Can you work these out from the model? Positions are in its coordinate system, mm. A direction names the side the tool comes from. Give positions to 0.01 mm unless a question says otherwise; leave off trailing zeros. Order: outer loops, then holes, each group sorted by start corner. A loop starts at its lowest first (then second) coordinate and runs counter-clockwise, first axis right, second up. Notation, with made-up numbers: M -36.5,75 L 18.5,75 A17 ccw 18.5,101 Z; hole C 62,50.5 d7. An arc over 180 degrees is marked long. Answer as a JSON object with one key per item and string values.
```python
from build123d import *

# Parameters (mm, degrees)
EXTRUDE_1_DEPTH          = 9.7
CUT_EXTRUDE_2_DEPTH      = 32.520737269
FILLET_3_R               = 0.5
CUT_EXTRUDE_5_DEPTH      = 32.353102755
CUT_EXTRUDE_5_DEPTH_BACK = 3.2
SKETCH_18_R              = 1
CUT_EXTRUDE_6_DEPTH      = 31.515193795


with BuildPart() as part:
    # 草图1 → 凸台-拉伸1 (new body)
    with BuildSketch(Plane.XY):
        with BuildLine():
            Line((-21, 14.94880858), (21, 14.94880858))
            Line((21, 14.94880858), (23.5, 14.94880858))
            Line((23.5, 14.94880858), (26, -1.615739558))
            ThreePointArc((26, -1.615739558), (0, 0), (-26, -1.615739558))
            Line((-26, -1.615739558), (-23.5, 14.94880858))
            Line((-23.5, 14.94880858), (-21, 14.94880858))
        make_face()
    extrude(amount=EXTRUDE_1_DEPTH)

    # 草图10 → 切除-拉伸2 (cut, through all)
    with BuildSketch(Plane.XY.offset(9.7)):
        Polygon((26, -1.615739558), (20.914837438, 15.00313582), (23.5, 14.94880858), align=None)
    cut_extrude_2 = extrude(amount=-CUT_EXTRUDE_2_DEPTH, mode=Mode.SUBTRACT)

    # 镜向1: 切除-拉伸2 across plane
    add(cut_extrude_2.mirror(Plane(origin=(0, 0, 0), x_dir=(0, 0, 1), z_dir=(1, 0, 0))), mode=Mode.SUBTRACT)

    # 圆角3
    fillet_3_edges = [part.edges().sort_by_distance(p)[0] for p in [
        (26, -1.615739558, 4.85),
        (-26, -1.615739558, 4.85),
        (0, 14.94880858, 0),
        (23.465730438, 6.666534511, 0),
        (20.931460876, 14.94880858, 4.85),
        (-23.465730438, 6.666534511, 0),
        (-20.931460876, 14.94880858, 4.85),
    ]]
    fillet(fillet_3_edges, radius=FILLET_3_R)

    # 草图17 → 切除-拉伸5 (cut, two sides: drawn at the far end of the back side and taken through both)
    with BuildSketch(Plane.XY.offset(9.7).offset(-CUT_EXTRUDE_5_DEPTH_BACK)):
        Polygon((-10, 103.759816228), (-10, 14.94880858), (-10, 4.94880858), (10, 4.94880858), (10, 14.94880858), (10, 103.759816228), (10, 281.381831522), (-10, 281.381831522), align=None)
    extrude(amount=CUT_EXTRUDE_5_DEPTH + CUT_EXTRUDE_5_DEPTH_BACK, mode=Mode.SUBTRACT)

    # 草图18 → 切除-拉伸6 (cut, through all)
    with BuildSketch(Plane.XY.offset(6.5)):
        with Locations((-6, 8.94880858)):
            Circle(SKETCH_18_R)
        with Locations((6, 8.94880858)):
            Circle(SKETCH_18_R)
    extrude(amount=-CUT_EXTRUDE_6_DEPTH, mode=Mode.SUBTRACT)


solid = part.part
```
1) Thinking about a two-plate mould opening in X: for faces 3 (the face through (0, 3, 9.7)), 4 (the face through (23.44, 6.75, 5.16)), 5 (the face through (0, 0, 5)), 6 (the face through (0, 4.949, 8)), which applies, pulls with the +X half, pulls with the -X half, needs draft (parallel to the pull), parting line crosses it, or undercut?
Results found:
{"face 3": "needs draft", "face 4": "pulls with the +X half", "face 5": "undercut", "face 6": "undercut"}
2) I want a section at B-B on z = 1.25. Write out the boundary of the cut face in (x, y), and give its area (3 significant figures).
Results found:
{"outline": "M -25.77,-0.88 A0.5 ccw -25.24,-1.52 A210 cw 25.24,-1.52 A0.5 ccw 25.77,-0.88 L 21.04,14.6 A0.5 ccw 20.56,14.95 L -20.56,14.95 A0.5 ccw -21.04,14.6 Z; hole C -6,8.95 d2; hole C 6,8.95 d2", "area": "715 mm²"}
3) I'm going to push flat-ended pins straight in: pin 1 Ø1 at (y, z) = (3, 2) entering from +X; pin 2 Ø1.6 at (y, z) = (11, 8) entering from +X; pin 3 Ø5 at (x, z) = (11.5, 7) entering from -Y; pin 4 Ø1.8 at (x, y) = (6, 8.95) entering from -Z. Where does each tip first touch, or does it pass through?
Results found:
{"pin 1": "stops at x = 24.74", "pin 2": "stops at x = 22.38", "pin 3": "stops at y = -0.47", "pin 4": "passes through"}
4) I need wall thicknesses on L1, parallel to X at y = 9.5, z = 1.25; L2, parallel to Y at x = -6, z = 4.25; L3, parallel to Z at x = 4, y = 7. Which ranges of each line are inside material? Lowest first, please.
Results found:
{"L1": "x = -22.6 to -6.83, -5.17 to 5.17, 6.83 to 22.6", "L2": "y = -0.09 to 7.95, 9.95 to 14.95", "L3": "z = 0 to 6.5"}
5) I want a section at A-A on x = -6. Write out the boundary of the cut face in (y, z).
Results found:
{"outline": "M -0.09,0 L 7.95,0 L 7.95,6.5 L 4.95,6.5 L 4.95,9.7 L -0.09,9.7 Z; M 9.95,0 L 14.45,0 A0.5 ccw 14.95,0.5 L 14.95,6.5 L 9.95,6.5 Z"}
6) For faces 1 (the face through (-6.74, 9.62, 3.3)), 2 (the face through (10, 10, 8)), which set-ups out of +Z, -Z, +X, -X, +Y, -Y let a thin tool reach every point of the face, with its end or its side?
Results found:
{"face 1": "+Z, -Z", "face 2": "+Z, +Y"}
7) I want a section at D-D on x = 9.5. Write out the boundary of the cut face in (y, z) (3 decimals), and give its area (3 significant figures).
Results found:
{"outline": "M -0.215,0 L 14.449,0 A0.5 ccw 14.949,0.5 L 14.949,6.5 L 4.949,6.5 L 4.949,9.7 L -0.215,9.7 Z", "area": "115 mm²"}
8) I want a section at C-C on z = 9. Write out the boundary of the cut face in (x, y).
Results found:
{"outline": "M -25.77,-0.88 A0.5 ccw -25.24,-1.52 A210 cw 25.24,-1.52 A0.5 ccw 25.77,-0.88 L 21.04,14.6 A0.5 ccw 20.56,14.95 L 10,14.95 L 10,4.95 L -10,4.95 L -10,14.95 L -20.56,14.95 A0.5 ccw -21.04,14.6 Z"}
